Verification items for the finished model (mm, model axes). Round coordinates to 2 decimals unless told otherwise and drop trailing zeros. Loops run counter-clockwise (first coordinate to the right, second up) from the corner with the lowest first, then second, coordinate; pieces in that order, holes last.
from build123d import *

# Parameters (mm, degrees)
SKETCH_1_W      = 32
SKETCH_1_H      = 25
EXTRUDE_1_DEPTH = 6
FILLET_1_R      = 3


with BuildPart() as part:
    # 草图1 → 凸台-拉伸1 (new body)
    with BuildSketch(Plane(origin=(0, 0, 0), x_dir=(1, 0, 0), z_dir=(0, 1, 0))):
        Rectangle(SKETCH_1_W, SKETCH_1_H)
    extrude(amount=EXTRUDE_1_DEPTH)

    # 圆角1
    fillet_1_edges = [part.edges().sort_by_distance(p)[0] for p in [
        (0, 0, -12.5),
        (0, 6, -12.5),
        (0, 6, 12.5),
        (0, 0, 12.5),
    ]]
    fillet(fillet_1_edges, radius=FILLET_1_R - 0.0001)  # a hair under: the kernel refuses the full size


solid = part.part
1. Scan lines: L1, parallel to Z at x = -8, y = 4.65; L2, parallel to Z at x = -1.5, y = 3.1; L3, parallel to Y at x = -3.5, z = 11.5. Record each from-to range of solid material in increasing order.
2. Section check C-C (y = 1.4). Enter the section's corners in (x, z), then the cut area to 3 significant figures.
3. Gauge pin test, flat ends, axial feed: P1, Ø1, axis at x = 0.5, y = 4, coming from the +Z side; P2, Ø1, axis at x = -0.5, y = 1, coming from the +Z side. Record the tip position at first contact, or that the pin passes through.
4. Section check B-B (y = 5). Enter the section's corners in (x, z).
Taken from the geometry:
1. L1: z = -12.01 to 12.01
1. L2: z = -12.5 to 12.5
1. L3: y = 0.76 to 5.24
2. outline: (-16, -12.04) - (16, -12.04) - (16, 12.04) - (-16, 12.04) - close
2. area: 770 mm2
3. P1: stops at z = 12.46
3. P2: stops at z = 12.1
4. outline: (-16, -11.74) - (16, -11.74) - (16, 11.74) - (-16, 11.74) - close
